```python
from build123d import *

# Parameters (mm, degrees)
BASPROSKE_W            = 3.175
BASPROSKE_H            = 9
TOOTHCUT_DEPTH         = 14.117950488
TEETHCUTS_COUNT        = 16
TEETHCUTS_ANGLE        = 337.5
BORSKE_R               = 1
BORE_DEPTH             = 50.0016256
CUT_EXTRUDE2_START     = -3.175
CUT_EXTRUDE2_OUTLINE_R = 1.4
CUT_EXTRUDE2_DEPTH     = 3.175


# Read off the part's stored shape, not the designer's step: Cut-Extrude2
with BuildPart() as part:
    # BasProSke → Base-Revolve (revolve)
    with BuildSketch(Plane(origin=(0, 0, 0), x_dir=(1, 0, 0), z_dir=(0, 1, 0)), mode=Mode.PRIVATE) as base_revolve_sk:
        with Locations((1.5875, 4.5)):
            Rectangle(BASPROSKE_W, BASPROSKE_H)
    revolve(base_revolve_sk.sketch.rotate(Axis((-10, 0, 0), (1, 0, 0)), 180), axis=Axis((-10, 0, 0), (1, 0, 0)))

    # TooCutSke → ToothCut (cut, through all)
    with BuildSketch(Plane(origin=(0, 0, 0), x_dir=(0, 0, -1), z_dir=(1, 0, 0))):
        with BuildLine():
            ThreePointArc((0.523792937, 6.728643397), (0, 6.749), (-0.523792937, 6.728643397))
            ThreePointArc((-0.523792937, 6.728643397), (-0.828704482, 7.90962059), (-1.553355277, 8.890721711))
            ThreePointArc((-1.553355277, 8.890721711), (0, 9.0254), (1.553355277, 8.890721711))
            ThreePointArc((1.553355277, 8.890721711), (0.828704482, 7.90962059), (0.523792937, 6.728643397))
        make_face()
    toothcut = extrude(amount=TOOTHCUT_DEPTH, mode=Mode.SUBTRACT)

    # TeethCuts: ToothCut ×16 about axis
    teethcuts_axis = Axis((-10, 0, 0), (1, 0, 0))
    for i in range(1, TEETHCUTS_COUNT):
        add(toothcut.rotate(teethcuts_axis, i * TEETHCUTS_ANGLE / (TEETHCUTS_COUNT - 1)), mode=Mode.SUBTRACT)

    # BorSke → Bore (cut, symmetric)
    with BuildSketch(Plane(origin=(0, 0, 0), x_dir=(0, 0, -1), z_dir=(1, 0, 0))):
        with Locations(Location((0, 0, 0), (0, 0, 180))):
            Circle(BORSKE_R)
    extrude(amount=BORE_DEPTH, both=True, mode=Mode.SUBTRACT)

    # Cut-Extrude2 outline → Cut-Extrude2 (cut)
    with BuildSketch(Plane(origin=(0, 0.498479729, -127.163742786), x_dir=(0, -0.6257802276580691, -0.779999427353774), z_dir=(-1, 0, 0)).offset(CUT_EXTRUDE2_START)):
        with Locations((-98.465111461, 75.484141115)):
            Circle(CUT_EXTRUDE2_OUTLINE_R)
        with Locations((-99.286304129, 84.446598512)):
            Circle(CUT_EXTRUDE2_OUTLINE_R)
    extrude(amount=CUT_EXTRUDE2_DEPTH, mode=Mode.SUBTRACT)


solid = part.part
```
Verification items for the finished model (mm, model axes). A direction names the side the tool comes from. Coordinates: 2 decimals unless noted, no trailing zeros. Order: outer loops, then holes, each group sorted by start corner. A loop starts at its lowest first (then second) coordinate and runs counter-clockwise, first axis right, second up. Notation, with made-up numbers: (70, 14) - (77, 14) arc R7 ccw to (77, 20) - close; hole circle Ø9 at (60.25, 73). An arc over 180 degrees is marked (long way). Return JSON: item names as keys, results as strings.
(1) Go/stop test with a flat-tipped pin: pin 1 (1 mm diameter, centred on x = 2, z = 6, fed in from +Y). Record where the tip stops, or that it passes through.
Filled sheet:
{"pin 1": "stops at y = 5.1"}
(2) Thickness scan on line 1 along Z through (x, y) = (0.7, 6.5); line 2 along Z through (x, y) = (0.65, -7.5). Record the ranges inside material, lowest first.
Filled sheet:
{"line 1": "z = -5.1 to -3.35, -2.12 to 2.12, 3.35 to 5.1", "line 2": "z = -4.97 to -4.55, -2.27 to -0.67, 0.67 to 2.27, 4.55 to 4.97"}
(3) Mould release check, pull along Y, two halves, no side actions. Record for faces 1 (the cylindrical face through (1.57, -6.75, 0.01)), 2 (the cylindrical face through (1.57, 0.83, 7.91)): pulls with the +Y half, pulls with the -Y half, needs draft (parallel to the pull), parting line crosses it, or undercut.
Filled sheet:
{"face 1": "pulls with the -Y half", "face 2": "undercut"}
(4) Section check C-C, the plane z = 7. Record the cut outline in (x, y) (3 decimals).
Filled sheet:
{"outline": "(0, -5.181) - (3.175, -5.181) - (3.175, -3.803) - (0, -3.803) - close; (0, -2.232) - (3.175, -2.232) - (3.175, -0.552) - (0, -0.552) - close; (0, 0.552) - (3.175, 0.552) - (3.175, 2.232) - (0, 2.232) - close; (0, 3.803) - (3.175, 3.803) - (3.175, 5.181) - (0, 5.181) - close"}
(5) Section check D-D, the plane x = 1.2. Give the number of separate pieces and of enclosed holes in the cut face, and give its area (3 significant figures).
Filled sheet:
{"separate pieces": "1", "enclosed holes": "3", "area": "176 mm^2"}
(6) Access from +Z, -Z, +X, -X, +Y, -Y to the whole of each face (thin tool, end or side, straight path). Record for faces 3 (the cylindrical face through (1.565, -6.232, 2.59)), 4 (the cylindrical face through (1.57, -0.83, -7.91)).
Filled sheet:
{"face 3": "+X, -X", "face 4": "-Z, +X, -X"}
(7) Section check A-A, the plane y = 0. Record the cut outline in (x, z) (3 decimals).
Filled sheet:
{"outline": "(0, -6.749) - (3.175, -6.749) - (3.175, -1) - (0, -1) - close; (0, 1) - (3.175, 1) - (3.175, 6.749) - (0, 6.749) - close"}
